The listing builds one solid part. Answer for the finished solid, in the listing's coordinates (mm). A direction names the side the tool comes from. Round coordinates to 2 decimals unless told otherwise and drop trailing zeros. Write each loop counter-clockwise with the first axis right and the second up, starting at its lowest first coordinate (ties: lowest second). Pieces come first, ordered by that corner, then holes. Notation, with made-up numbers: M 88.25,55 L 125.25,55 A22 ccw 125.25,83 Z; hole C -5,27.5 d11. An arc over 180 degrees is marked long. Put each result on its own line as item: value. Start each with the question number.
Autodesk Inventor part; units mm, degrees
ref_plane "Work Plane1" through (32.075, -15, -15) normal (1, 0, 0) x (0, 1, 0)
ref_plane "Start Plane" through (0, 0, 0) normal (1, 0, 0) x (0, 1, 0)
ref_plane "XZ Plane" through (0, 0, 0) normal (0, 1, 0) x (-1, 0, 0)
sketch "Main Sketch" plane through (0, 0, 0) normal (0, 0, 1) x (1, 0, 0)
  line L0 (0, 0) -> (37.5, 0)
  line L1 (0, 0) -> (0, 1.205)
  line L2 (0, 1.205) -> (3, 1.205)
  line L3 (3, 1.205) -> (3, 3)
  line L4 (7.5, 3) -> (7.5, 1.25)
  line L5 (3, 3) -> (7.5, 3)
  line L6 (7.5, 1.25) -> (10.5, 1.25)
  line L7 (10.5, 1.25) -> (10.5, 3)
  line L8 (37.5, 3) -> (37.5, 0)
  line L9 (10.5, 3) -> (37.5, 3)
  dimension "d3" = 2.41
  dimension "d4" = 6
  dimension "d5" = 2.5
  dimension "d6" = 6
revolve "Revolution1" add sketch "Main Sketch" angle 360 about axis through (0, 0, 0) along (1, 0, 0)
sketch "Sketch3" plane through (37.5, 0, 0) normal (1, 0, 0) x (0, 0, -1)
  circle A0 centre (0, 0) radius 3
  circle A1 centre (0, 0) radius 3
  line L0 (2.45, 1.7313) -> (2.45, -1.7313)
  dimension "d8" = 5.45
extrude "Extrusion1" cut sketch "Sketch3" against normal blind 11.5 contours A0 L0 picked at (2.5504, -0.3987)
ref_plane "Work Plane1" through (32.075, -15, -15) normal (1, 0, 0) x (0, 1, 0)
sketch "Sketch5" plane through (37.5, 0, 0) normal (1, 0, 0) x (0, 0, -1)
  line L0 (2.45, -1.7313) -> (2.45, 1.7313)
  arc A0 (2.45, 1.7313) -> (2.45, -1.7313) centre (0, 0) ccw
extrude "Extrusion3" cut sketch "Sketch5" against normal blind 2.7
sketch "Sketch6" plane through (0, 0, 0) normal (-1, 0, 0) x (0, 0, 1)
  circle A0 centre (0, 0) radius 1.205
  circle A1 centre (0, 0) radius 1.205
  circle A2 centre (0, 0) radius 3
extrude "Extrusion4" cut sketch "Sketch6" against normal up to surface (3 mm away) contours A0 | A2
equation "\"Length\" = 37.5"
properties part number "Shaft" material "Steel"
Item 1: Determine the mould class of faces 4 (the cylindrical face through (9.02, -0.27, -1.22)), 5 (the flat face through (3, 0, 0)), 6 (the cylindrical face through (5, -3, 0)) for opening direction X: released by +X, released by -X, zero draft, split by the parting line, or undercut.
Item 2: Flat-ended cylindrical pins translate along their axes: pin 1 (3 mm diameter, centred on x = 32, y = 0, fed in from -Z); pin 2 (1 mm diameter, centred on x = 28.5, y = -2, fed in from +Z). Find the tip coordinate at first contact, or state that the pin passes through.
Item 3: Section A-A (y = 2.6) is taken. Give the vertices of the cut face in (x, z).
Item 4: Section C-C (x = 9.5) is taken. Give the vertices of the cut face in (y, z).
Item 5: Which of the six approach directions +Z, -Z, +X, -X, +Y, -Y give full straight-line access (tool end or side, diameter ignored) to faces 1 (the flat face through (10.5, 1, -1)), 2 (the cylindrical face through (23, 0, 3)), 3 (the flat face through (30, 0, -2.45))?
Item 6: Section B-B (z = 0) is taken. Give the vertices of the cut face in (x, y).
Item 7: Section D-D (z = -1.55) is taken. Give the vertices of the cut face in (x, y).
Item 8: Consider line 1 along X through (y, z) = (-1.15, 1.4); line 2 along X through (y, z) = (-1.1, -2.6); line 3 along Y through (x, z) = (30, 0.5). Determine where each line is inside the solid, lowest interval first. Write a range as [from, to].
Output values:
1. face 4: undercut
1. face 5: released by -X
1. face 6: zero draft
2. pin 1: stops at z = -2.45
2. pin 2: stops at z = 2.6
3. outline: M 3,-1.5 L 7.5,-1.5 L 7.5,1.5 L 3,1.5 Z; M 10.5,-1.5 L 34.8,-1.5 L 34.8,1.5 L 10.5,1.5 Z
4. outline: C 0,0 d2.5
5. face 1: none
5. face 2: +X, -X
5. face 3: -Z, +X, +Y, -Y
6. outline: M 3,-3 L 7.5,-3 L 7.5,-1.25 L 10.5,-1.25 L 10.5,-3 L 34.8,-3 L 34.8,3 L 10.5,3 L 10.5,1.25 L 7.5,1.25 L 7.5,3 L 3,3 Z
7. outline: M 3,-2.57 L 7.5,-2.57 L 7.5,2.57 L 3,2.57 Z; M 10.5,-2.57 L 34.8,-2.57 L 34.8,2.57 L 10.5,2.57 Z
8. line 1: x = [3, 7.5], [10.5, 34.8]
8. line 2: x = [3, 7.5], [10.5, 26]
8. line 3: y = [-2.96, 2.96]
